from build123d import *

# Parameters (mm, degrees)
SKETCH1_W           = 38
SKETCH1_H           = 78
BOSS_EXTRUDE1_DEPTH = 10
SKETCH2_R           = 7.65
CUT_EXTRUDE1_DEPTH  = 88.338422244
SKETCH3_R           = 1.75
CUT_EXTRUDE2_DEPTH  = 88.338422244


with BuildPart() as part:
    # Sketch1 → Boss-Extrude1 (new body)
    with BuildSketch(Plane.XY):
        with Locations((19, 39)):
            Rectangle(SKETCH1_W, SKETCH1_H)
    extrude(amount=BOSS_EXTRUDE1_DEPTH)

    # Sketch2 → Cut-Extrude1 (cut, through all)
    with BuildSketch(Plane.ZY):
        with Locations((0, 69)):
            Circle(SKETCH2_R)
        with Locations((0, 9)):
            Circle(SKETCH2_R)
    extrude(amount=-CUT_EXTRUDE1_DEPTH, mode=Mode.SUBTRACT)

    # Sketch3 → Cut-Extrude2 (cut, through all)
    with BuildSketch(Plane(origin=(0, 0, 0), x_dir=(-1, 0, 0), z_dir=(0, 0, -1))):
        with Locations((-36.2, 39)):
            Circle(SKETCH3_R)
        with Locations((-1.8, 39)):
            Circle(SKETCH3_R)
    extrude(amount=-CUT_EXTRUDE2_DEPTH, mode=Mode.SUBTRACT)


solid = part.part
Verification items for the finished model (mm, model axes). Round coordinates to 2 decimals unless told otherwise and drop trailing zeros. Loops run counter-clockwise (first coordinate to the right, second up) from the corner with the lowest first, then second, coordinate; pieces in that order, holes last. Notation, with made-up numbers: (-6.75, -33) - (33.25, -33) arc R33 cw to (33.25, -3) - close; hole circle Ø1 at (-21.75, 51.25). An arc over 180 degrees is marked (long way). Answer in a Markdown table with one row per item. Add a question column.
Q1. Section check A-A on x = 36.2. Enter the section's corners in (y, z).
Q2. Release check for a two-part mould opening along Y. For faces 1 (the face through (2.18, 37.29, 4.93)), 2 (the face through (18.73, 68.83, 7.65)), 3 (the face through (19, 78, 5)), 4 (the face through (0, 38, 6)) record: pulls with the +Y half, pulls with the -Y half, needs draft (parallel to the pull), parting line crosses it, or undercut.
Q3. Section check C-C on z = 6.25. Enter the section's corners in (x, y), plus the area to 3 significant figures.
Q4. Section check B-B on z = 2.25. Enter the section's corners in (x, y), plus the area to 3 significant figures.
Q5. Section check D-D on x = 18.5. Enter the section's corners in (y, z).
Q6. Material ranges on line 1 (Y direction, x = 36.2, z = 6.5); line 2 (Y direction, x = 18, z = 5.75); line 3 (Y direction, x = 18, z = 2.75), recorded low to high.
Found:
| question | item | result |
|---|---|---|
| 1 | outline | (0, 0) - (1.35, 0) arc R7.65 cw to (16.65, 0) - (37.25, 0) - (37.25, 10) - (0, 10) - close; (40.75, 0) - (61.35, 0) arc R7.65 cw to (76.65, 0) - (78, 0) - (78, 10) - (40.75, 10) - close |
| 2 | face 1 | undercut |
| 2 | face 2 | undercut |
| 2 | face 3 | pulls with the +Y half |
| 2 | face 4 | needs draft |
| 3 | outline | (0, 0) - (38, 0) - (38, 4.59) - (0, 4.59) - close; (0, 13.41) - (38, 13.41) - (38, 64.59) - (0, 64.59) - close; (0, 73.41) - (38, 73.41) - (38, 78) - (0, 78) - close; hole circle Ø3.5 at (1.8, 39); hole circle Ø3.5 at (36.2, 39) |
| 3 | area | 2,270 mm² |
| 4 | outline | (0, 0) - (38, 0) - (38, 1.69) - (0, 1.69) - close; (0, 16.31) - (38, 16.31) - (38, 61.69) - (0, 61.69) - close; (0, 76.31) - (38, 76.31) - (38, 78) - (0, 78) - close; hole circle Ø3.5 at (1.8, 39); hole circle Ø3.5 at (36.2, 39) |
| 4 | area | 1,830 mm² |
| 5 | outline | (0, 0) - (1.35, 0) arc R7.65 cw to (16.65, 0) - (61.35, 0) arc R7.65 cw to (76.65, 0) - (78, 0) - (78, 10) - (0, 10) - close |
| 6 | line 1 | y = 0 to 4.97, 13.03 to 37.25, 40.75 to 64.97, 73.03 to 78 |
| 6 | line 2 | y = 0 to 3.95, 14.05 to 63.95, 74.05 to 78 |
| 6 | line 3 | y = 0 to 1.86, 16.14 to 61.86, 76.14 to 78 |
